Study the drawing (mm; zero at the part's minimum x, y, z) and answer. Round coordinates to 2 decimals unless told otherwise and drop trailing zeros. Write each loop counter-clockwise with the first axis right and the second up, starting at its lowest first coordinate (ties: lowest second). Pieces come first, ordered by that corner, then holes.
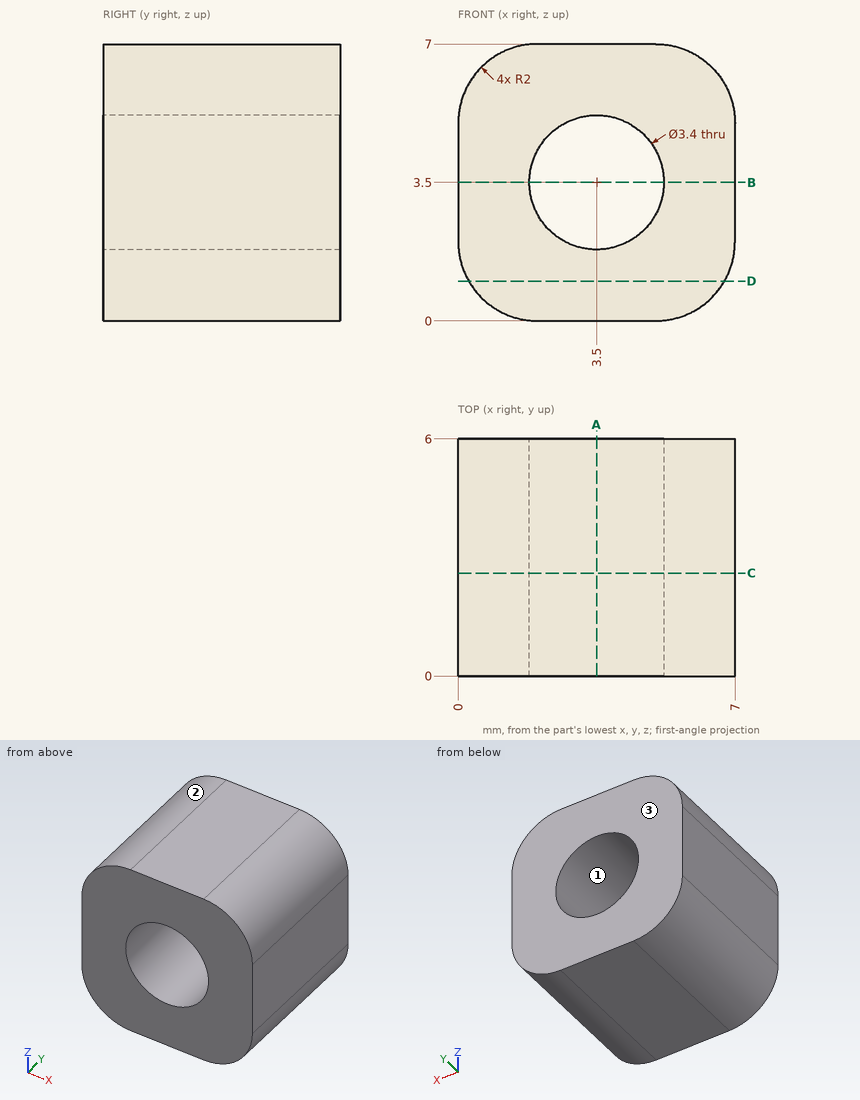
Q1. Find section D-D (z = 1). Determine the outline of the cut face in (x, y), plus the area to 3 significant figures.
Q2. The mould has two halves that part along X. Classify the marked faces 1, 2 and 3: +X half, -X half, draft (parallel to the pull), parting line (faces both ways), or undercut.
Q3. Find the intervals of material crossed by L1, parallel to Z at x = 3.5, y = 2.75; L2, parallel to Z at x = 4, y = 5.1, in increasing order.
Q4. Find section C-C (y = 2.6). Determine the outline of the cut face in (x, z), plus the area to 3 significant figures.
Q5. Find section A-A (x = 3.5). Determine the outline of the cut face in (y, z), plus the area to 3 significant figures.
Q6. Find section B-B (z = 3.5). Determine the outline of the cut face in (x, y).
Report:
1. outline: (0.27, 0) - (6.73, 0) - (6.73, 6) - (0.27, 6) - close
1. area: 38.8 mm2
2. face 1: undercut
2. face 2: -X half
2. face 3: draft
3. L1: z = 0 to 1.8, 5.2 to 7
3. L2: z = 0 to 1.88, 5.12 to 7
4. outline: (0, 2) arc R2 ccw to (2, 0) - (5, 0) arc R2 ccw to (7, 2) - (7, 5) arc R2 ccw to (5, 7) - (2, 7) arc R2 ccw to (0, 5) - close; hole circle Ø3.4 at (3.5, 3.5)
4. area: 36.5 mm2
5. outline: (0, 0) - (6, 0) - (6, 1.8) - (0, 1.8) - close; (0, 5.2) - (6, 5.2) - (6, 7) - (0, 7) - close
5. area: 21.6 mm2
6. outline: (0, 0) - (1.8, 0) - (1.8, 6) - (0, 6) - close; (5.2, 0) - (7, 0) - (7, 6) - (5.2, 6) - close
